```python
from build123d import *

# Parameters (mm, degrees)
SM_BASE_FLANGE_1_DEPTH = 4
M4X0_251_D             = 3.75
M4X0_251_DEPTH         = 9.25
M4X0_251_TIP           = 1.126613661


# Sheet-metal steps are written as plain solids
with BuildPart() as part:
    # Sketch 1 → Базовая кромка1 (new body)
    with BuildSketch(Plane.XY):
        with BuildLine():
            Line((-14.5, -17.5), (14.5, -17.5))
            ThreePointArc((14.5, -17.5), (16.621320344, -16.621320344), (17.5, -14.5))
            Line((17.5, -14.5), (17.5, 14.5))
            ThreePointArc((17.5, 14.5), (16.621320344, 16.621320344), (14.5, 17.5))
            Line((14.5, 17.5), (-14.5, 17.5))
            ThreePointArc((-14.5, 17.5), (-16.621320344, 16.621320344), (-17.5, 14.5))
            Line((-17.5, 14.5), (-17.5, -14.5))
            ThreePointArc((-17.5, -14.5), (-16.621320344, -16.621320344), (-14.5, -17.5))
        make_face()
    extrude(amount=SM_BASE_FLANGE_1_DEPTH)

    # Отверстие обработанное метчиком M4x0.251
    with Locations(Plane(origin=(0, 0, 0), x_dir=(-1, 0, 0), z_dir=(0, 0, -1))):
        with Locations((-10.960155108, 10.960155108), (10.960155108, 10.960155108), (10.960155108, -10.960155108), (-10.960155108, -10.960155108)):
            Hole(M4X0_251_D / 2, depth=M4X0_251_DEPTH)
            with Locations((0, 0, -(M4X0_251_DEPTH + M4X0_251_TIP / 2))):  # 118° drill point
                Cone(0, M4X0_251_D / 2, M4X0_251_TIP, mode=Mode.SUBTRACT)


solid = part.part
```
CAD build for the part. Positions are in the model's coordinates, mm. Coordinates: 2 decimals unless noted, no trailing zeros. Write each loop counter-clockwise with the first axis right and the second up, starting at its lowest first coordinate (ties: lowest second). Pieces come first, ordered by that corner, then holes. Notation, with made-up numbers: (-24.5, 85) -> (-12.5, 85) arc R9 cw to (-12.5, 93) -> close; hole circle Ø2 at (-11, 84.25). An arc over 180 degrees is marked (long way). Use CSV: the item, a comma, the result in double quotes. Start each with the question number.
Item 1: Wall check: probe 1 along X at (y, z) = (-10, 2.15); probe 2 along Y at (x, z) = (-10.5, 0.9); probe 3 along X at (y, z) = (-12, 0.3). Give the ranges that are in metal, low to high.
Item 2: Band-saw the part on B-B, the plane x = 12. Write the cut outline in (y, z), plus the area to 3 significant figures.
Item 3: Band-saw the part on A-A, the plane z = 2.85. Write the cut outline in (x, y) (3 decimals).
Item 4: Drop a flat-ended pin along its axis: P1, Ø6, axis at x = 6.5, y = -9, coming from the -Z side. Give the stop position or say it passes through.
Item 5: Two-plate mould, pull along X, no slides. Class faces 1 (the cylindrical face through (-16.6, 16.64, 1.97)), 2 (the cylindrical face through (-11.2, 12.82, 2.03)), 3 (the cylindrical face through (16.6, -16.64, 1.97)), 4 (the cylindrical face through (9.087, -10.878, 2.028)): +X half, -X half, draft (parallel to the pull), parting line (faces both ways), or undercut.
Response values:
1,probe 1,"x = -17.5 to -12.57, -9.35 to 9.35, 12.57 to 17.5"
1,probe 2,"y = -17.5 to -12.78, -9.14 to 9.14, 12.78 to 17.5"
1,probe 3,"x = -17.5 to -12.52, -9.4 to 9.4, 12.52 to 17.5"
2,outline,"(-17.5, 0) -> (-12.52, 0) -> (-12.52, 4) -> (-17.5, 4) -> close; (-9.4, 0) -> (9.4, 0) -> (9.4, 4) -> (-9.4, 4) -> close; (12.52, 0) -> (17.5, 0) -> (17.5, 4) -> (12.52, 4) -> close"
2,area,"115 mm2"
3,outline,"(-17.5, -14.5) arc R3 ccw to (-14.5, -17.5) -> (14.5, -17.5) arc R3 ccw to (17.5, -14.5) -> (17.5, 14.5) arc R3 ccw to (14.5, 17.5) -> (-14.5, 17.5) arc R3 ccw to (-17.5, 14.5) -> close; hole circle Ø3.75 at (-10.96, -10.96); hole circle Ø3.75 at (-10.96, 10.96); hole circle Ø3.75 at (10.96, -10.96); hole circle Ø3.75 at (10.96, 10.96)"
4,P1,"stops at z = 0"
5,face 1,"-X half"
5,face 2,"undercut"
5,face 3,"+X half"
5,face 4,"undercut"
